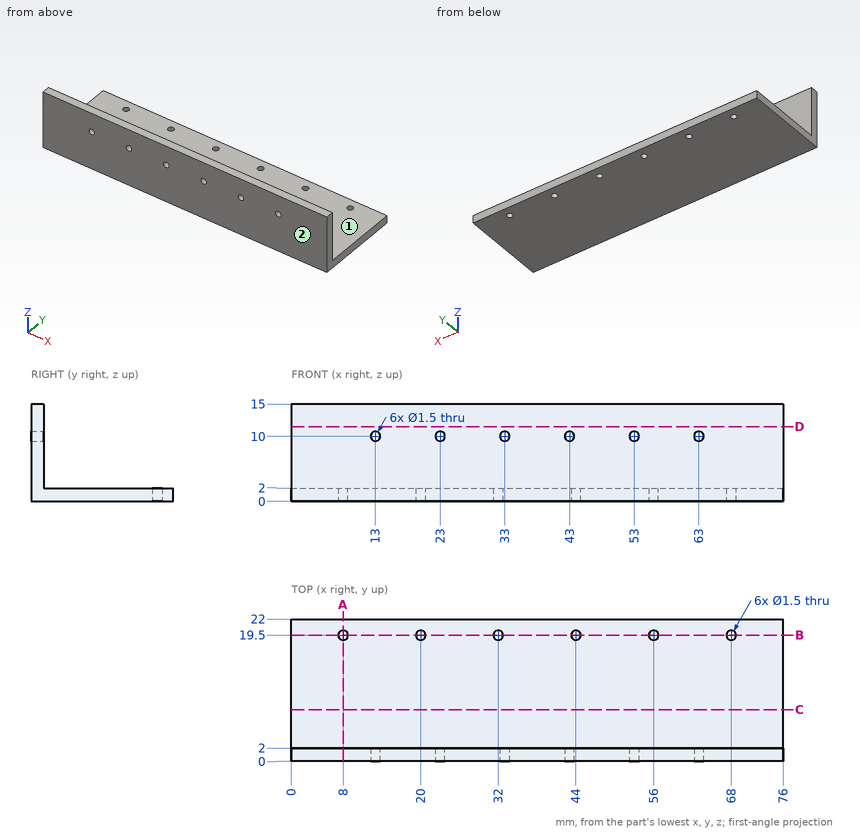
Job drawing, mm, ordinate dimensions from the low corner. One solid piece. A direction names the side the tool comes from. Round coordinates to 2 decimals unless told otherwise and drop trailing zeros. Order: outer loops, then holes, each group sorted by start corner. A loop starts at its lowest first (then second) coordinate and runs counter-clockwise, first axis right, second up. Notation, with made-up numbers: (84.25, 52) - (112.25, 52) arc R9 cw to (112.25, 62) - close; hole circle Ø10 at (20.5, 77). An arc over 180 degrees is marked (long way). Use CSV: the item, a comma, the result in double quotes. Start each with the question number.
1) Pin check, flat tips, straight feed: pin 1 Ø6 at (x, y) = (29, 11) entering from +Z; pin 2 Ø1.4 at (x, y) = (56, 19.5) entering from -Z; pin 3 Ø4 at (x, z) = (41.5, 7) entering from +Y. Stop position of each tip, or through.
2) Saw through at C-C (y = 8). List the corners of the cut face in (x, z).
3) Wall check: L1, parallel to Y at x = 44, z = 1.05; L2, parallel to Z at x = 63, y = 1.3; L3, parallel to Y at x = 55.5, z = 11.75. Give the ranges that are in metal, low to high. Write a range as [from, to].
4) Saw through at A-A (x = 8). List the corners of the cut face in (y, z), and give its area (3 significant figures).
5) Saw through at B-B (y = 19.5). List the corners of the cut face in (x, z), and give its area (3 significant figures).
6) Tool access for the marked faces 1 and 2: list every direction of +Z, -Z, +X, -X, +Y, -Y with a clear straight run to the whole face (end or side of a thin tool).
Values follow:
1,pin 1,"stops at z = 2"
1,pin 2,"passes through"
1,pin 3,"stops at y = 2"
2,outline,"(0, 0) - (76, 0) - (76, 2) - (0, 2) - close"
3,L1,"y = [0, 18.75], [20.25, 22]"
3,L2,"z = [0, 9.25], [10.75, 15]"
3,L3,"y = [0, 2]"
4,outline,"(0, 0) - (18.75, 0) - (18.75, 2) - (2, 2) - (2, 15) - (0, 15) - close; (20.25, 0) - (22, 0) - (22, 2) - (20.25, 2) - close"
4,area,"67.0 mm2"
5,outline,"(0, 0) - (7.25, 0) - (7.25, 2) - (0, 2) - close; (8.75, 0) - (19.25, 0) - (19.25, 2) - (8.75, 2) - close; (20.75, 0) - (31.25, 0) - (31.25, 2) - (20.75, 2) - close; (32.75, 0) - (43.25, 0) - (43.25, 2) - (32.75, 2) - close; (44.75, 0) - (55.25, 0) - (55.25, 2) - (44.75, 2) - close; (56.75, 0) - (67.25, 0) - (67.25, 2) - (56.75, 2) - close; (68.75, 0) - (76, 0) - (76, 2) - (68.75, 2) - close"
5,area,"134 mm2"
6,face 1,"+Z, +X, -X, +Y"
6,face 2,"+Z, -Z, +X, -X, -Y"
